The listing builds one solid part. Answer for the finished solid, in the listing's coordinates (mm). Coordinates: 2 decimals unless noted, no trailing zeros. Loops run counter-clockwise (first coordinate to the right, second up) from the corner with the lowest first, then second, coordinate; pieces in that order, holes last. Notation, with made-up numbers: (74.25, 88) - (100.25, 88) arc R30 ccw to (100.25, 126) - close; hole circle Ø7 at (-2, 34.5). An arc over 180 degrees is marked (long way). Put each result on its own line as item: value.
```python
from build123d import *

# Parameters (mm, degrees)
F0_W     = 201.676
F0_H     = 153.924
F1_DEPTH = 3.175
F2_W     = 76.2
F2_H     = 50.8
F3_DEPTH = 3.176
F4_W     = 176.276
F4_H     = 9.525
F5_DEPTH = 3.176
F6_R     = 5.08


with BuildPart() as f1:
    # F0 (on Front) → F1 (new body)
    with BuildSketch(Plane.XZ):
        Rectangle(F0_W, F0_H)
    extrude(amount=F1_DEPTH)

    # F2 (on face) → F3 (cut, through all)
    with BuildSketch(Plane.XZ.offset(3.175)):
        with Locations((-50.038, 43.688)):
            Rectangle(F2_W, F2_H)
        with Locations((51.562, -18.2245)):
            Rectangle(F2_W, F2_H)
    extrude(amount=-F3_DEPTH, mode=Mode.SUBTRACT)

    # F4 (on face) → F5 (cut, through all)
    with BuildSketch(Plane.XZ.offset(3.175)):
        with Locations((0, -65.8495)):
            Rectangle(F4_W, F4_H)
    extrude(amount=-F5_DEPTH, mode=Mode.SUBTRACT)

    # F6
    f6_edges = [f1.edges().sort_by_distance(p)[0] for p in [
        (100.838, -1.5875, 76.962),
        (100.838, -1.5875, -76.962),
        (-100.838, -1.5875, 76.962),
        (-100.838, -1.5875, -76.962),
    ]]
    fillet(f6_edges, radius=F6_R)


solid = f1.part
```
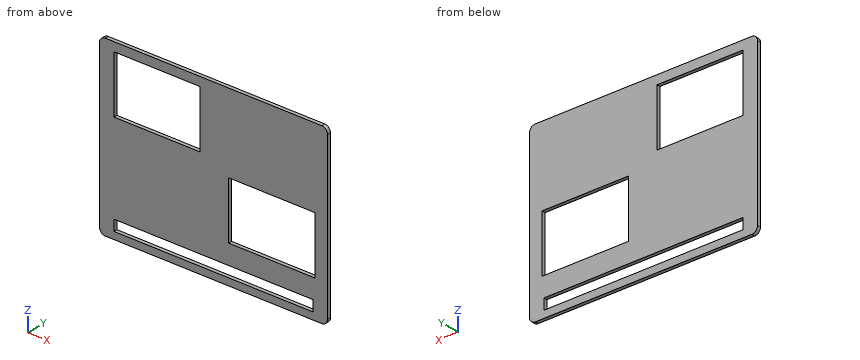
1) The part is cut by section A-A (x = 84). Give the vertices of the cut face in (y, z) (1 decimal), and give its area (3 significant figures).
Found:
outline: (-3.2, -77) - (0, -77) - (0, -70.6) - (-3.2, -70.6) - close; (-3.2, -61.1) - (0, -61.1) - (0, -43.6) - (-3.2, -43.6) - close; (-3.2, 7.2) - (0, 7.2) - (0, 77) - (-3.2, 77) - close
area: 297 mm^2
2) Straight lines are drawn through the part: L1, parallel to Z at x = -78.5, y = -0.5; L2, parallel to Z at x = 37, y = -1.5; L3, parallel to X at y = -2.4, z = 1. For each, find the intervals that lie inside material, in ascending order. Write a range as [from, to].
Found:
L1: z = [-76.96, -70.61], [-61.09, 18.29], [69.09, 76.96]
L2: z = [-76.96, -70.61], [-61.09, -43.62], [7.18, 76.96]
L3: x = [-100.84, 13.46], [89.66, 100.84]
3) The part is cut by section B-B (z = 42). Give the vertices of the cut face in (x, y) (3 decimals), and give its area (3 significant figures).
Found:
outline: (-100.838, -3.175) - (-88.138, -3.175) - (-88.138, 0) - (-100.838, 0) - close; (-11.938, -3.175) - (100.838, -3.175) - (100.838, 0) - (-11.938, 0) - close
area: 398 mm^2
4) The part is cut by section C-C (y = -0.75). Give the vertices of the cut face in (x, z), and give its area (3 significant figures).
Found:
outline: (-100.84, -71.88) arc R5.08 ccw to (-95.76, -76.96) - (95.76, -76.96) arc R5.08 ccw to (100.84, -71.88) - (100.84, 71.88) arc R5.08 ccw to (95.76, 76.96) - (-95.76, 76.96) arc R5.08 ccw to (-100.84, 71.88) - close; hole (-88.14, -70.61) - (88.14, -70.61) - (88.14, -61.09) - (-88.14, -61.09) - close; hole (-88.14, 18.29) - (-11.94, 18.29) - (-11.94, 69.09) - (-88.14, 69.09) - close; hole (13.46, -43.62) - (89.66, -43.62) - (89.66, 7.18) - (13.46, 7.18) - close
area: 21,600 mm^2
